Source: CAD feature listing. Evaluate the final solid. Frame: model axes, mm. Face numbers are marked on the shaded views. A direction names the side the tool comes from. Round coordinates to 2 decimals unless told otherwise and drop trailing zeros. Order: outer loops, then holes, each group sorted by start corner. A loop starts at its lowest first (then second) coordinate and runs counter-clockwise, first axis right, second up. Notation, with made-up numbers: (-4, -26.75) - (4, -26.75) arc R16 ccw to (4, -1.75) - close; hole circle Ø11 at (-36, 76). An arc over 180 degrees is marked (long way). Put each result on its own line as item: value. Start each with the question number.
1) Section B-B on x = 12.7. Output: boundary loops of the cut face in (y, z) (3 decimals), then the cut area to 3 significant figures.
2) Section D-D on y = 0.5. Output: boundary loops of the cut face in (x, z) (3 decimals).
3) Access query for the marked faces 1 and 2. Directions: +Z, -Z, +X, -X, +Y, -Y. A direction counts if a zero-diameter tool reaches every point of the face in a straight line with its end or side. Return the directions, or none.
4) Section C-C on z = 45.96. State how many separate pieces and enclosed holes the cut face has, then the cut area to 3 significant figures.
5) Contact query for flat-ended pins moving along their axis: P1, Ø3, axis at x = 15, y = 4.5, coming from the +Z side; P2, Ø4, axis at y = 7.5, z = 37.5, coming from the +X side (3 decimals); P3, Ø3, axis at x = 14.5, z = 28, coming from the +Y side (3 decimals). Output: stop coordinate, or through.
6) Line query: probe 1 along Z at (x, y) = (12.7, 0.65) (3 decimals); probe 2 along Y at (x, z) = (2.3, 20.56); probe 3 along Z at (x, y) = (14, 1.25). Output: solid intervals per line, ascending. Write a range as [from, to].
7) Section A-A on y = 8. Output: boundary loops of the cut face in (x, z) (1 decimal).
```python
from build123d import *

# Parameters (mm, degrees)
BOSS_EXTRUDE1_DEPTH = 50.8
SKETCH2_R           = 1.5875
CUT_EXTRUDE1_DEPTH  = 10
SKETCH5_R           = 3.175
CUT_EXTRUDE2_DEPTH  = 6.35


with BuildPart() as part:
    # Sketch1 → Boss-Extrude1 (new body)
    with BuildSketch(Plane.XY):
        Polygon((0, 0), (0, 11), (3.175, 11), (3.175, 3.175), (19.05, 3.175), (19.05, 0), align=None)
    extrude(amount=BOSS_EXTRUDE1_DEPTH)

    # Sketch2 → Cut-Extrude1 (cut)
    with BuildSketch(Plane(origin=(3.175, 0, 0), x_dir=(0, 0, -1), z_dir=(1, 0, 0))):
        with Locations((-45.96, 8)):
            Circle(SKETCH2_R)
        with Locations((-30.24, 8)):
            Circle(SKETCH2_R)
        with Locations((-20.56, 8)):
            Circle(SKETCH2_R)
        with Locations((-4.84, 8)):
            Circle(SKETCH2_R)
    extrude(amount=-CUT_EXTRUDE1_DEPTH, mode=Mode.SUBTRACT)

    # Sketch5 → Cut-Extrude2 (cut)
    with BuildSketch(Plane(origin=(0, 3.175, 0), x_dir=(1, 0, 0), z_dir=(0, 1, 0))):
        with Locations((12.7, -6.35)):
            Circle(SKETCH5_R)
        with Locations((12.7, -44.45)):
            Circle(SKETCH5_R)
    extrude(amount=-CUT_EXTRUDE2_DEPTH, mode=Mode.SUBTRACT)


solid = part.part
```
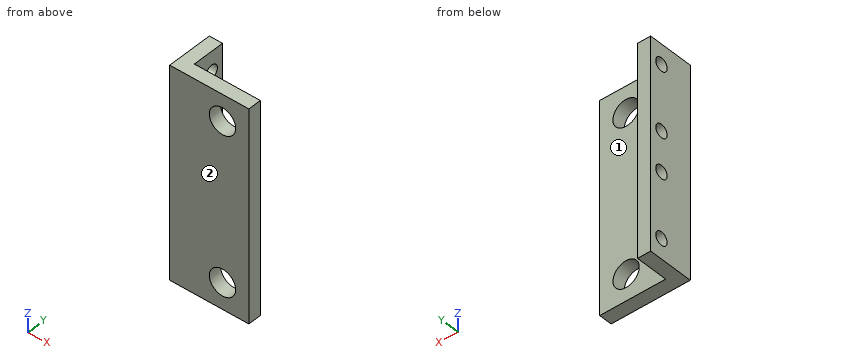
Answer sheet:
1. outline: (0, 0) - (3.175, 0) - (3.175, 3.175) - (0, 3.175) - close; (0, 9.525) - (3.175, 9.525) - (3.175, 41.275) - (0, 41.275) - close; (0, 47.625) - (3.175, 47.625) - (3.175, 50.8) - (0, 50.8) - close
1. area: 121 mm^2
2. outline: (0, 0) - (19.05, 0) - (19.05, 50.8) - (0, 50.8) - close; hole circle Ø6.35 at (12.7, 6.35); hole circle Ø6.35 at (12.7, 44.45)
3. face 1: +Z, -Z, +X, +Y
3. face 2: +Z, -Z, +X, -X, -Y
4. separate pieces: 3
4. enclosed holes: 0
4. area: 57.5 mm^2
5. P1: z = 50.8
5. P2: x = 3.175
5. P3: y = 3.175
6. probe 1: [0, 3.175], [9.525, 41.275], [47.625, 50.8]
6. probe 2: [0, 6.41], [9.59, 11]
6. probe 3: [0, 3.45], [9.25, 41.55], [47.35, 50.8]
7. outline: (0, 0) - (3.2, 0) - (3.2, 3.3) - (0, 3.3) - close; (0, 6.4) - (3.2, 6.4) - (3.2, 19) - (0, 19) - close; (0, 22.1) - (3.2, 22.1) - (3.2, 28.7) - (0, 28.7) - close; (0, 31.8) - (3.2, 31.8) - (3.2, 44.4) - (0, 44.4) - close; (0, 47.5) - (3.2, 47.5) - (3.2, 50.8) - (0, 50.8) - close
